CAD build for the part. Positions are in the model's coordinates, mm. Face numbers are marked on the shaded views. Round coordinates to 2 decimals unless told otherwise and drop trailing zeros. Write each loop counter-clockwise with the first axis right and the second up, starting at its lowest first coordinate (ties: lowest second). Pieces come first, ordered by that corner, then holes. Notation, with made-up numbers: (69, 85.5) -> (110, 85.5) arc R26 cw to (110, 120.5) -> close; hole circle Ø2 at (-21.75, -32). An arc over 180 degrees is marked (long way). Answer in a Markdown table with one row per item. Add a question column.
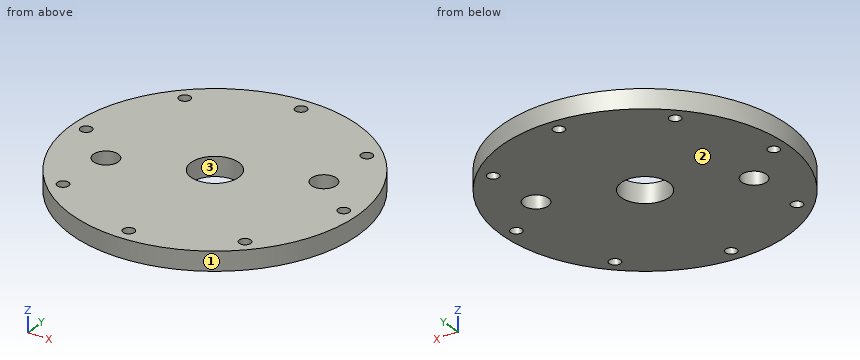
```python
from build123d import *

# Parameters (mm, degrees)
CROQUIS1_R              = 75
CROQUIS1_R_2            = 3
CROQUIS1_R_3            = 12.5
SALIENTE_EXTRUIR1_DEPTH = 10
CROQUIS2_R              = 6.5
CORTAR_EXTRUIR1_DEPTH   = 10


with BuildPart() as part:
    # Croquis1 → Saliente-Extruir1 (new body)
    with BuildSketch(Plane.XY):
        Circle(CROQUIS1_R)
        with Locations((0, 67.5)):
            Circle(CROQUIS1_R_2, mode=Mode.SUBTRACT)
        with Locations((47.72970773, 47.72970773)):
            Circle(CROQUIS1_R_2, mode=Mode.SUBTRACT)
        with Locations((67.5, 0)):
            Circle(CROQUIS1_R_2, mode=Mode.SUBTRACT)
        with Locations((47.72970773, -47.72970773)):
            Circle(CROQUIS1_R_2, mode=Mode.SUBTRACT)
        with Locations((0, -67.5)):
            Circle(CROQUIS1_R_2, mode=Mode.SUBTRACT)
        with Locations((-47.72970773, -47.72970773)):
            Circle(CROQUIS1_R_2, mode=Mode.SUBTRACT)
        with Locations((-67.5, 0)):
            Circle(CROQUIS1_R_2, mode=Mode.SUBTRACT)
        with Locations((-47.72970773, 47.72970773)):
            Circle(CROQUIS1_R_2, mode=Mode.SUBTRACT)
        Circle(CROQUIS1_R_3, mode=Mode.SUBTRACT)
    extrude(amount=SALIENTE_EXTRUIR1_DEPTH)

    # Croquis2 → Cortar-Extruir1 (cut)
    with BuildSketch(Plane.XY.offset(10)):
        with Locations((45.570866947, 17.316425315)):
            Circle(CROQUIS2_R)
        with Locations((-45.570866947, -17.316425315)):
            Circle(CROQUIS2_R)
    extrude(amount=-CORTAR_EXTRUIR1_DEPTH, mode=Mode.SUBTRACT)


solid = part.part
```
Item 1: Saw through at B-B on x = 0. Give the cut face in (y, z), then the cut area to 3 significant figures.
Item 2: Saw through at A-A on y = 67.5. Give the cut face in (x, z), then the cut area to 3 significant figures.
Item 3: Saw through at D-D on z = 3.5. Count the separate pieces of the cut face and the enclosed holes in it, then the cut area to 3 significant figures.
Item 4: Drill centre lines: probe 1 along Y at (x, z) = (0, 2.75); probe 2 along X at (y, z) = (-54, 2.75); probe 3 along X at (y, z) = (20.5, 6). Where is each one in solid material? Low to high.
Item 5: Pin check, flat tips, straight feed: pin 1 (5 mm diameter, centred on x = 38, z = 6, fed in from -Y); pin 2 (2 mm diameter, centred on y = -50.5, z = 3.5, fed in from -X); pin 3 (6 mm diameter, centred on y = 34.5, z = 2.5, fed in from -X). Stop position of each tip, or through.
Item 6: Two-plate mould, pull along X, no slides. Class the marked faces 1, 2 and 3: +X half, -X half, draft (parallel to the pull), parting line (faces both ways), or undercut.
Recorded:
| question | item | result |
|---|---|---|
| 1 | outline | (-75, 0) -> (-70.5, 0) -> (-70.5, 10) -> (-75, 10) -> close; (-64.5, 0) -> (-12.5, 0) -> (-12.5, 10) -> (-64.5, 10) -> close; (12.5, 0) -> (64.5, 0) -> (64.5, 10) -> (12.5, 10) -> close; (70.5, 0) -> (75, 0) -> (75, 10) -> (70.5, 10) -> close |
| 1 | area | 1,130 mm2 |
| 2 | outline | (-32.69, 0) -> (-3, 0) -> (-3, 10) -> (-32.69, 10) -> close; (3, 0) -> (32.69, 0) -> (32.69, 10) -> (3, 10) -> close |
| 2 | area | 594 mm2 |
| 3 | separate pieces | 1 |
| 3 | enclosed holes | 11 |
| 3 | area | 16,700 mm2 |
| 4 | probe 1 | -75 to -70.5, -64.5 to -12.5, 12.5 to 64.5, 70.5 to 75 |
| 4 | probe 2 | -52.05 to 52.05 |
| 4 | probe 3 | -72.14 to 39.9, 51.24 to 72.14 |
| 5 | pin 1 | y = -66.07 |
| 5 | pin 2 | x = -56.34 |
| 5 | pin 3 | x = -68.06 |
| 6 | face 1 | parting line |
| 6 | face 2 | draft |
| 6 | face 3 | undercut |
